Build history of the part. All positions in model axes, mm. Face numbers are marked on the shaded views. A direction names the side the tool comes from. Give positions to 0.01 mm unless a question says otherwise; leave off trailing zeros. Order: outer loops, then holes, each group sorted by start corner. A loop starts at its lowest first (then second) coordinate and runs counter-clockwise, first axis right, second up. Notation, with made-up numbers: (10, 46) -> (33, 46) arc R34 ccw to (33, 79) -> close; hole circle Ø2 at (19.25, 63.25). An arc over 180 degrees is marked (long way). One line per item, written item: value. Start each with the question number.
(1) Probe line 1 (X direction, y = 22, z = 0); line 2 (Z direction, x = 0, y = 29.25); line 3 (Z direction, x = 0, y = 34.25). List the from-to ranges inside material, lowest first.
(2) Saw through at D-D on y = 16. Give the cut face in (x, z), plus the area to 3 significant figures.
(3) Saw through at C-C on x = 0. Give the cut face in (y, z), plus the area to 3 significant figures.
(4) Saw through at B-B on y = 28.5. Give the cut face in (x, z), plus the area to 3 significant figures.
(5) Pin check, flat tips, straight feed: pin 1 (6 mm diameter, centred on x = 6.5, z = 6.5, fed in from -Y); pin 2 (1 mm diameter, centred on x = -5, y = 39, fed in from -Z); pin 3 (8 mm diameter, centred on x = 0, z = 0, fed in from +Y); pin 4 (6 mm diameter, centred on x = 11.5, y = 35, fed in from +Z). Stop position of each tip, or through.
(6) Two-plate mould, pull along X, no slides. Class the marked faces 1, 2, 3 and 4: +X half, -X half, draft (parallel to the pull), parting line (faces both ways), or undercut.
(7) Saw through at A-A on z = 0. Give the cut face in (x, y).
(8) Which spindle directions (+Z, -Z, +X, -X, +Y, -Y) get a long thin tool onto all of the face, cutting with end or side? Do the marked faces 5 and 6. Say none if no direction does.
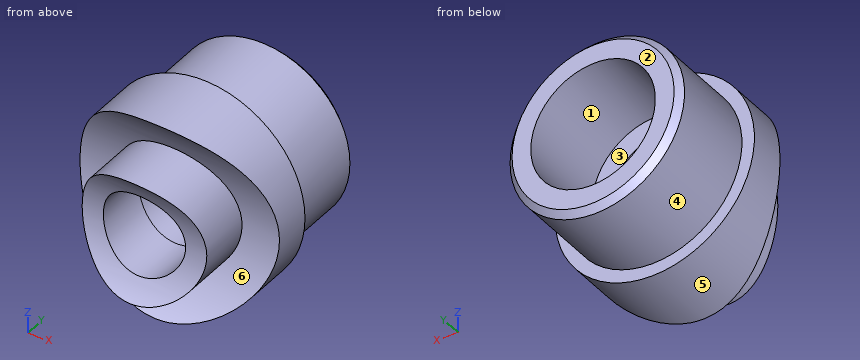
```python
from build123d import *

# Parameters (mm, degrees)
SKETCH1_R               = 16
SKETCH1_R_2             = 6.6
BOSS_EXTRUDE1_DEPTH     = 31
SKETCH2_R               = 14
SKETCH2_R_2             = 10
BOSS_EXTRUDE2_DEPTH     = 14.5
SKETCH3_R               = 25
CUT_EXTRUDE1_DEPTH      = 17
CUT_EXTRUDE1_DEPTH_BACK = 17
BOSS_EXTRUDE3_REACH     = 47.5
SKETCH4_R               = 10
SKETCH4_R_2             = 6.6
SKETCH5_R               = 16.7
CUT_EXTRUDE2_DEPTH      = 17.0000001
CUT_EXTRUDE2_DEPTH_BACK = 17.0000001
CHAMFER1_SIZE           = 1


with BuildPart() as part:
    # Sketch1 → Boss-Extrude1 (new body)
    with BuildSketch(Plane(origin=(0, 0, 0), x_dir=(1, 0, 0), z_dir=(0, 1, 0))):
        Circle(SKETCH1_R)
        Circle(SKETCH1_R_2, mode=Mode.SUBTRACT)
    extrude(amount=BOSS_EXTRUDE1_DEPTH)

    # Sketch2 → Boss-Extrude2 (add)
    with BuildSketch(Plane(origin=(0, 31, 0), x_dir=(1, 0, 0), z_dir=(0, 1, 0))):
        Circle(SKETCH2_R)
        Circle(SKETCH2_R_2, mode=Mode.SUBTRACT)
    extrude(amount=BOSS_EXTRUDE2_DEPTH)

    # Sketch3 → Cut-Extrude1 (cut, two sides)
    with BuildSketch(Plane(origin=(0, 0, 0), x_dir=(0, 0, -1), z_dir=(1, 0, 0))) as cut_extrude1_sk:
        Circle(SKETCH3_R)
    extrude(amount=CUT_EXTRUDE1_DEPTH, mode=Mode.SUBTRACT)
    extrude(cut_extrude1_sk.sketch, amount=-CUT_EXTRUDE1_DEPTH_BACK, mode=Mode.SUBTRACT)

    # Sketch4 → Boss-Extrude3 (add, up to next)
    with BuildSketch(Plane(origin=(0, 0, 0), x_dir=(1, 0, 0), z_dir=(0, 1, 0)), mode=Mode.PRIVATE) as boss_extrude3_sk1:
        Circle(SKETCH4_R)
        Circle(SKETCH4_R_2, mode=Mode.SUBTRACT)
    boss_extrude3_tool1 = extrude(boss_extrude3_sk1.sketch, amount=BOSS_EXTRUDE3_REACH, mode=Mode.PRIVATE) - part.part
    add(boss_extrude3_tool1.solids().sort_by_distance((-9.717157, 0, 0))[0])

    # Sketch5 → Cut-Extrude2 (cut, two sides)
    with BuildSketch(Plane(origin=(0, 0, 0), x_dir=(0, 0, -1), z_dir=(1, 0, 0))) as cut_extrude2_sk:
        Circle(SKETCH5_R)
    extrude(amount=CUT_EXTRUDE2_DEPTH, mode=Mode.SUBTRACT)
    extrude(cut_extrude2_sk.sketch, amount=-CUT_EXTRUDE2_DEPTH_BACK, mode=Mode.SUBTRACT)

    # Chamfer1
    chamfer1_edges = [part.edges().sort_by_distance(p)[0] for p in [
        (-14, 45.5, 0),
    ]]
    chamfer(chamfer1_edges, length=CHAMFER1_SIZE)


solid = part.part
```
Results below:
1. line 1: x = -10 to -6.6, 6.6 to 10
1. line 2: z = -16 to -6.6, 6.6 to 16
1. line 3: z = -14 to -10, 10 to 14
2. outline: (-8.78, -4.78) arc R10 ccw to (8.78, -4.78) -> (4.55, -4.78) arc R6.6 cw to (-4.55, -4.78) -> close; (-8.78, 4.78) -> (-4.55, 4.78) arc R6.6 cw to (4.55, 4.78) -> (8.78, 4.78) arc R10 ccw to start
2. area: 108 mm²
3. outline: (13.37, -10) -> (22.91, -10) arc R25 cw to (19.21, -16) -> (31, -16) -> (31, -14) -> (44.5, -14) -> (45.5, -13) -> (45.5, -10) -> (31, -10) -> (31, -6.6) -> (15.34, -6.6) arc R16.7 cw to start; (13.37, 10) arc R16.7 cw to (15.34, 6.6) -> (31, 6.6) -> (31, 10) -> (45.5, 10) -> (45.5, 13) -> (44.5, 14) -> (31, 14) -> (31, 16) -> (19.21, 16) arc R25 cw to (22.91, 10) -> close
3. area: 344 mm²
4. outline: circle Ø32 at (0, 0); hole circle Ø13.2 at (0, 0)
4. area: 667 mm²
5. pin 1: stops at y = 14.16
5. pin 2: stops at z = -13.26
5. pin 3: passes through
5. pin 4: stops at z = 11.12
6. face 1: undercut
6. face 2: draft
6. face 3: undercut
6. face 4: parting line
7. outline: (-16, 25) -> (-10, 25) -> (-10, 16.7) -> (-6.6, 16.7) -> (-6.6, 31) -> (-10, 31) -> (-10, 45.5) -> (-13, 45.5) -> (-14, 44.5) -> (-14, 31) -> (-16, 31) -> close; (6.6, 16.7) -> (10, 16.7) -> (10, 25) -> (16, 25) -> (16, 31) -> (14, 31) -> (14, 44.5) -> (13, 45.5) -> (10, 45.5) -> (10, 31) -> (6.6, 31) -> close
8. face 5: +Y, -Y
8. face 6: -Y
